Geometry: final body of the model. Coordinates: model frame, mm. A direction names the side the tool comes from. Give positions to 0.01 mm unless a question says otherwise; leave off trailing zeros. Write each loop counter-clockwise with the first axis right and the second up, starting at its lowest first coordinate (ties: lowest second). Pieces come first, ordered by that corner, then holes. Notation, with made-up numbers: M 80.25,-26 L 123.25,-26 A18 cw 123.25,-18 Z; hole C 44,-9 d10. An arc over 180 degrees is marked long. Answer as a JSON object with one key per item and string values.
from build123d import *

# Parameters (mm, degrees)
F0_R            = 28
F0_R_2          = 25
F1_DEPTH        = 15
F4_DEPTH        = 2.5
F4_COPIES_COUNT = 4


# Not quite as in the source:
# - a pattern or mirror of a feature is missing from the dataset's text; its kind, count and spacing are read off the source's solid


with BuildPart() as f1:
    # F0 (on Top) → F1 (new body)
    with BuildSketch(Plane.XY):
        Circle(F0_R)
        Circle(F0_R_2, mode=Mode.SUBTRACT)
    extrude(amount=F1_DEPTH)

    # F3 (on offset) → F4 (join, symmetric)
    with BuildSketch(Plane.XY.offset(7.5)):
        with BuildLine():
            ThreePointArc((0, 23), (5.9528380374, 22.2162940046), (11.5, 19.918584287))
            Line((11.5, 19.918584287), (12.5, 21.6506350946))
            ThreePointArc((12.5, 21.6506350946), (6.4704761276, 24.1481456572), (0, 25))
            Line((0, 25), (0, 23))
        make_face()
    f4 = extrude(amount=F4_DEPTH, both=True)

    # F4_copies: F4 ×4 about axis
    f4_copies_axis = Axis((0, 0, 0), (0, 0, 1))
    for i in range(1, F4_COPIES_COUNT):
        add(f4.rotate(f4_copies_axis, i * 360 / F4_COPIES_COUNT))


solid = f1.part
1) Cut plane B-B on y = -24. Return loops of the section in (x, z), and give its area (3 significant figures).
Geometry check:
{"outline": "M -14.42,0 L -7,0 L -7,5 L 0,5 L 0,10 L -7,10 L -7,15 L -14.42,15 Z; M 7,0 L 14.42,0 L 14.42,15 L 7,15 Z", "area": "258 mm2"}
2) Cut plane D-D on z = 3.25. Return loops of the section in (x, y).
Geometry check:
{"outline": "C 0,0 d56; hole C 0,0 d50"}
3) Set-up query: faces 5 (the flat face through (-11.99, -20.77, 7.54)), 6 (the flat face through (-23, 6, 10)), 7 (the flat face through (23, -6, 5)). Return all of +Z, -Z, +X, -X, +Y, -Y with unobstructed straight access to the full face (end or side cutting, diameter ignored); none if empty.
Geometry check:
{"face 5": "+Z, -Z", "face 6": "+Z", "face 7": "-Z"}
4) Line query: line 1 (Y direction, x = 0, z = 3.5); line 2 (Y direction, x = 18, z = 2); line 3 (X direction, y = -13.5, z = 6.5). Output: solid intervals per line, ascending. Write a range as from..to.
Geometry check:
{"line 1": "y = -28..-25, 25..28", "line 2": "y = -21.45..-17.35, 17.35..21.45", "line 3": "x = -24.53..-21.04, 21.04..24.53"}
5) Pull-direction query (X, two-part tool) for faces 1 (the flat face through (20.77, -11.99, 7.54)), 2 (the flat face through (11.99, 20.77, 7.54)), 3 (the flat face through (-11, 23, 0)), 4 (the cylindrical face through (25.865, -10.724, 7.395)); classes: pulls with the +X half, pulls with the -X half, needs draft (parallel to the pull), parting line crosses it, or undercut.
Geometry check:
{"face 1": "undercut", "face 2": "undercut", "face 3": "needs draft", "face 4": "parting line crosses it"}
6) Contact query for flat-ended pins moving along their axis: P1, Ø1, axis at x = 23.5, z = 7.5, coming from the +Y side; P2, Ø4, axis at x = -6, y = -22.5, coming from the -Z side; P3, Ø2.5, axis at x = -22, y = 3.5, coming from the -Z side; P4, Ø1, axis at y = 24, z = 7, coming from the -X side. Output: stop coordinate, or through.
Geometry check:
{"P1": "stops at y = 15.97", "P2": "stops at z = 0", "P3": "stops at z = 5", "P4": "stops at x = -15.22"}
7) Cut plane A-A on z = 8. Return loops of the section in (x, y).
Geometry check:
{"outline": "C 0,0 d56; hole M -25,0 A25 ccw -12.5,-21.65 L -11.5,-19.92 A23 ccw 0,-23 L 0,-25 A25 ccw 21.65,-12.5 L 19.92,-11.5 A23 ccw 23,0 L 25,0 A25 ccw 12.5,21.65 L 11.5,19.92 A23 ccw 0,23 L 0,25 A25 ccw -21.65,12.5 L -19.92,11.5 A23 ccw -23,0 Z"}
8) Cut plane C-C on x = 10. Return loops of the section in (y, z), and give its area (3 significant figures).
Geometry check:
{"outline": "M -26.15,0 L -22.91,0 L -22.91,15 L -26.15,15 Z; M 20.71,5 L 22.91,5 L 22.91,0 L 26.15,0 L 26.15,15 L 22.91,15 L 22.91,10 L 20.71,10 Z", "area": "108 mm2"}
